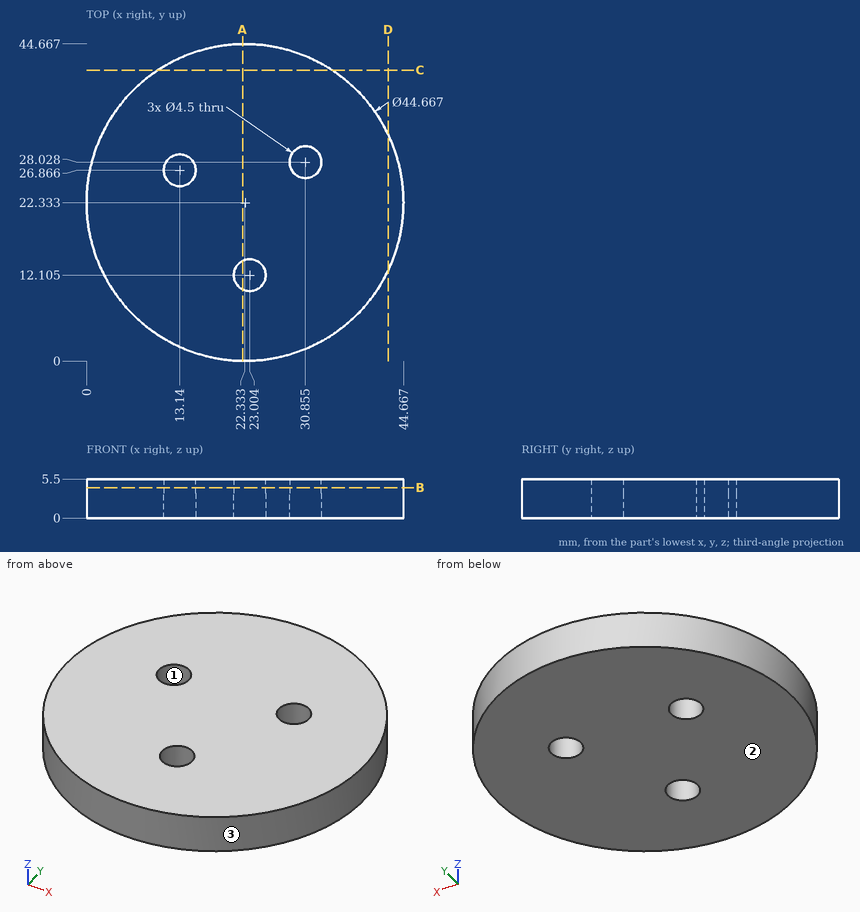
Design review of the part shown in the three views and the two pictorial views. Dimensions are in mm from the part's minimum x, y and z. Round coordinates to 2 decimals unless told otherwise and drop trailing zeros. Loops run counter-clockwise (first coordinate to the right, second up) from the corner with the lowest first, then second, coordinate; pieces in that order, holes last. Notation, with made-up numbers: M 87,65.25 L 102,65.25 A22 cw 102,83.25 Z; hole C -19,74.5 d2. An arc over 180 degrees is marked long. Write item = value, one per line.
Item 1: The part is to be moulded in two halves that separate along Y. For the marked faces 1, 2 and 3, say which applies: released by +Y, released by -Y, zero draft, split by the parting line, or undercut.
Return value:
face_1 = undercut
face_2 = zero draft
face_3 = split by the parting line
Item 2: Take a section at B-B on z = 4.3. State how many separate pieces and enclosed holes the cut face has, then the cut area to 3 significant figures.
Return value:
separate_pieces = 1
enclosed_holes = 3
area = 1,520 mm2
Item 3: For line 1 (X direction, y = 28, z = 2.5) (1 decimal); line 2 (X direction, y = 27.5, z = 2.2) (1 decimal); line 3 (X direction, y = 11.5, z = 2.35) (1 decimal), list the stretches that pass through material, from the lowest coordinate up. Write a range as [from, to].
Return value:
line_1 = [0.7, 11.2], [15.1, 28.6], [33.1, 43.9]
line_2 = [0.6, 11], [15.3, 28.7], [33, 44.1]
line_3 = [2.8, 20.8], [25.2, 41.9]
Item 4: Take a section at A-A on x = 22. Write out the cut boundary in (y, z) (1 decimal).
Return value:
outline = M 0,0 L 10.1,0 L 10.1,5.5 L 0,5.5 Z; M 14.1,0 L 44.7,0 L 44.7,5.5 L 14.1,5.5 Z
Item 5: Take a section at C-C on y = 41. Write out the cut boundary in (x, z) (1 decimal), then the cut area to 3 significant figures.
Return value:
outline = M 10.1,0 L 34.6,0 L 34.6,5.5 L 10.1,5.5 Z
area = 135 mm2
Item 6: Take a section at D-D on x = 42.5. Write out the cut boundary in (y, z).
Return value:
outline = M 12.74,0 L 31.93,0 L 31.93,5.5 L 12.74,5.5 Z
Item 7: Insertion check: P1, Ø1.5, axis at x = 12.5, z = 3, coming from the -Y side; P2, Ø4, axis at x = 13.14, y = 26.87, coming from the +Z side; P3, Ø1, axis at y = 29.5, z = 5, coming from the +X side. Each pin has a flat end and moves straight along its axis. Give the tip position at first contact, or say it passes through.
Return value:
P1 = 1.93
P2 = through
P3 = 43.65
